For this review, take the finished solid that the model builds, in its own axes (mm). A direction names the side the tool comes from. Coordinates: 2 decimals unless noted, no trailing zeros. Loops run counter-clockwise (first coordinate to the right, second up) from the corner with the lowest first, then second, coordinate; pieces in that order, holes last.
1. To check wall thickness, follow probe 1 along X at (y, z) = (32, -10.5) (3 decimals); probe 2 along Z at (x, y) = (0, 21); probe 3 along Y at (x, z) = (0, -19.4). State the ranges of each line that lie inside material, in increasing order.
2. Take a section at C-C, the plane y = 42.5. State the section outline as (x, z) points (1 decimal), then the cut area to 3 significant figures.
3. Mouldability with a two-part tool opening along Y and no side actions: class faces 1 (the face through (2, 0, -18)), 2 (the face through (-1, 35, -20.638)), 3 (the face through (0.72, 7.19, -19.03)) as pulls with the +Y half, pulls with the -Y half, needs draft (parallel to the pull), parting line crosses it, or undercut.
4. Take a section at B-B, the plane y = 57. State the section outline as (x, z) points (1 decimal), then the cut area to 3 significant figures.
5. Machinability: for faces 4 (the face through (-25.4, 22, 0)), 5 (the face through (0, 50.8, 0)), 6 (the face through (0, 22, -17.462)), 7 (the face through (25.4, 22, 0)), which of the approach directions +Z, -Z, +X, -X, +Y, -Y give a long, thin tool a straight path to every point of the face, cutting with its end or side? Answer none if there is none.
6. Take a section at A-A, the plane x = 0. State the section outline as (y, z) points, then the cut area to 3 significant figures.
7. Clearance check with flat-ended pins moving along their axes: P1, Ø1.5, axis at x = -16.5, z = 15, coming from the -Y side; P2, Ø10.5, axis at y = 30, z = -3.5, coming from the +X side; P3, Ø9.5, axis at y = 20.5, z = -3, coming from the -X side. State where each tip first meets the part, or that it passes through.
8. Take a section at D-D, the plane x = -19. State the section outline as (y, z) points, then the cut area to 3 significant figures.
```python
from build123d import *

# Parameters (mm, degrees)
F0_W     = 50.8
F0_H     = 41.275
F0_W_2   = 44.45
F0_H_2   = 34.925
F1_DEPTH = 44.45
F3_DEPTH = 20.6375
F5_DEPTH = 82.551
F7_D     = 7.9375
F8_R     = 6.35
F9_R     = 5.08
F11_D    = 11.1125


with BuildPart() as f1:
    # F0 (on Front) → F1 (new body)
    with BuildSketch(Plane.XZ):
        Rectangle(F0_W, F0_H)
        Rectangle(F0_W_2, F0_H_2, mode=Mode.SUBTRACT)
    extrude(amount=-F1_DEPTH)

    # F2 (on Top) → F3 (join, symmetric)
    with BuildSketch(Plane.XY):
        Polygon((41.275, 44.45), (41.275, 107.95), (34.925, 107.95), (34.925, 101.6), (34.925, 50.8), (-34.925, 50.8), (-34.925, 101.6), (-34.925, 107.95), (-41.275, 107.95), (-41.275, 44.45), align=None)
    extrude(amount=F3_DEPTH, both=True)

    # F4 (on face) → F5 (cut, through all)
    with BuildSketch(Plane(origin=(-41.275, 0, 0), x_dir=(0, -1, 0), z_dir=(-1, 0, 0))):
        with BuildLine():
            Line((-107.95, -20.6375), (-87.3125, -20.6375))
            ThreePointArc((-87.3125, -20.6375), (-101.9054161967, -14.5929161967), (-107.95, 0))
            Line((-107.95, 0), (-107.95, -20.6375))
        make_face()
        with BuildLine():
            ThreePointArc((-107.95, 0), (-101.9054161967, 14.5929161967), (-87.3125, 20.6375))
            Line((-87.3125, 20.6375), (-107.95, 20.6375))
            Line((-107.95, 20.6375), (-107.95, 0))
        make_face()
    extrude(amount=-F5_DEPTH, mode=Mode.SUBTRACT)

    # F7 (through all)
    with Locations(Plane(origin=(-41.275, 0, 0), x_dir=(0, -1, 0), z_dir=(-1, 0, 0))):
        with Locations((-87.3125, 0)):
            Hole(F7_D / 2)

    # F8
    f8_edges = [f1.edges().sort_by_distance(p)[0] for p in [
        (-41.275, 44.45, 0),
        (41.275, 44.45, 0),
    ]]
    fillet(f8_edges, radius=F8_R)

    # F9
    f9_edges = [f1.edges().sort_by_distance(p)[0] for p in [
        (-25.4, 22.225, 20.6375),
        (25.4, 22.225, 20.6375),
        (25.4, 22.225, -20.6375),
        (-25.4, 22.225, -20.6375),
    ]]
    fillet(f9_edges, radius=F9_R)

    # F11 (through all)
    with Locations(Plane(origin=(0, 0, -20.6375), x_dir=(1, 0, 0), z_dir=(0, 0, -1))):
        with Locations((0, -12.7)):
            Hole(F11_D / 2)


solid = f1.part
```
Results list:
1. probe 1: x = -25.4 to -22.225, 22.225 to 25.4
1. probe 2: z = -20.64 to -17.46, 17.46 to 20.64
1. probe 3: y = 0 to 7.14, 18.26 to 50.8
2. outline: (-25.4, -15.6) arc R5.1 ccw to (-20.3, -20.6) - (20.3, -20.6) arc R5.1 ccw to (25.4, -15.6) - (25.4, 15.6) arc R5.1 ccw to (20.3, 20.6) - (-20.3, 20.6) arc R5.1 ccw to (-25.4, 15.6) - close; hole (-22.2, -17.5) - (22.2, -17.5) - (22.2, 17.5) - (-22.2, 17.5) - close
2. area: 522 mm2
3. face 1: pulls with the -Y half
3. face 2: needs draft
3. face 3: undercut
4. outline: (-41.3, -20.6) - (-34.9, -20.6) - (-34.9, 20.6) - (-41.3, 20.6) - close; (34.9, -20.6) - (41.3, -20.6) - (41.3, 20.6) - (34.9, 20.6) - close
4. area: 524 mm2
5. face 4: +Z, -Z, -X, -Y
5. face 5: +Z, -Z, +Y
5. face 6: -Y
5. face 7: +Z, -Z, +X, -Y
6. outline: (0, -20.64) - (7.14, -20.64) - (7.14, -17.46) - (0, -17.46) - close; (0, 17.46) - (7.14, 17.46) - (7.14, 20.64) - (0, 20.64) - close; (18.26, -20.64) - (50.8, -20.64) - (50.8, 20.64) - (18.26, 20.64) - (18.26, 17.46) - (44.45, 17.46) - (44.45, -17.46) - (18.26, -17.46) - close
6. area: 474 mm2
7. P1: stops at y = 44.45
7. P2: stops at x = 25.4
7. P3: stops at x = -25.4
8. outline: (0, -20.64) - (50.8, -20.64) - (50.8, 20.64) - (0, 20.64) - (0, 17.46) - (44.45, 17.46) - (44.45, -17.46) - (0, -17.46) - close
8. area: 544 mm2
